Build history of the part. All positions in model axes, mm. Give positions to 0.01 mm unless a question says otherwise; leave off trailing zeros. Loops run counter-clockwise (first coordinate to the right, second up) from the corner with the lowest first, then second, coordinate; pieces in that order, holes last. Notation, with made-up numbers: (5, -15.75) -> (30, -15.75) arc R14 cw to (30, -4.75) -> close; hole circle Ø5 at (0, -25.75). An arc over 180 degrees is marked (long way). Answer as a JSON object with one key per item and string values. Group by question number.
from build123d import *

# Parameters (mm, degrees)
F1_DEPTH = 4
F2_R     = 0.5
F4_D     = 4


with BuildPart() as f1:
    # F0 (on Top) → F1 (new body)
    with BuildSketch(Plane.XY):
        Polygon((-15, -10), (15, -10), (15, 10), (0, 30), (-15, 10), align=None)
    extrude(amount=F1_DEPTH)

    # F2
    f2_edges = [f1.edges().sort_by_distance(p)[0] for p in [
        (15, 10, 2),
        (15, -10, 2),
        (0, 30, 2),
        (-15, 10, 2),
        (-15, -10, 2),
    ]]
    fillet(f2_edges, radius=F2_R)

    # F4 (through all)
    with Locations(Plane(origin=(0, 0, 0), x_dir=(1, 0, 0), z_dir=(0, 0, -1))):
        with Locations((7.5, 0), (-7.5, 0)):
            Hole(F4_D / 2)


solid = f1.part
(1) Probe line 1 along Y through (x, z) = (-11.25, 2.2); line 2 along Y through (x, z) = (8, 3.5); line 3 along Y through (x, z) = (7, 2.85). List the from-to ranges inside material, lowest first. Write a range as [from, to].
(2) Pull direction X, two halves, no side cores. Call faces 1 (the cylindrical face through (9.498, -0.088, 2.028)), 2 (the flat face through (0, 6, 0)), 3 (the flat face through (15, 0, 2)): pulls with the +X half, pulls with the -X half, needs draft (parallel to the pull), parting line crosses it, or undercut.
(3) Saw through at C-C on x = -7.5. List the corners of the cut face in (y, z).
(4) Saw through at D-D on y = 24. List the corners of the cut face in (x, z).
(5) Saw through at B-B on y = 0. List the corners of the cut face in (x, z).
(6) Saw through at A-A on z = 0.5. List the corners of the cut face in (x, y).
(7) Pin check, flat tip, straight feed: pin 1 (1 mm diameter, centred on y = 13.5, z = 2.5, fed in from +X). Stop position of the tip, or through.
Calculated:
{
 "1": {"line 1": "y = [-10, 15]", "line 2": "y = [-10, -1.94], [1.94, 19.33]", "line 3": "y = [-10, -1.94], [1.94, 20.67]"},
 "2": {"face 1": "undercut", "face 2": "needs draft", "face 3": "pulls with the +X half"},
 "3": {"outline": "(-10, 0) -> (-2, 0) -> (-2, 4) -> (-10, 4) -> close; (2, 0) -> (20, 0) -> (20, 4) -> (2, 4) -> close"},
 "4": {"outline": "(-4.5, 0) -> (4.5, 0) -> (4.5, 4) -> (-4.5, 4) -> close"},
 "5": {"outline": "(-15, 0) -> (-9.5, 0) -> (-9.5, 4) -> (-15, 4) -> close; (-5.5, 0) -> (5.5, 0) -> (5.5, 4) -> (-5.5, 4) -> close; (9.5, 0) -> (15, 0) -> (15, 4) -> (9.5, 4) -> close"},
 "6": {"outline": "(-15, -9.5) arc R0.5 ccw to (-14.5, -10) -> (14.5, -10) arc R0.5 ccw to (15, -9.5) -> (15, 9.83) arc R0.5 ccw to (14.9, 10.13) -> (0.4, 29.47) arc R0.5 ccw to (-0.4, 29.47) -> (-14.9, 10.13) arc R0.5 ccw to (-15, 9.83) -> close; hole circle Ø4 at (-7.5, 0); hole circle Ø4 at (7.5, 0)"},
 "7": {"pin 1": "stops at x = 12.75"}
}
